The drawing under review shows one solid part. Ordinate dimensions are in mm from its lowest x, y, z. A direction names the side the tool comes from. Round coordinates to 2 decimals unless told otherwise and drop trailing zeros. Write each loop counter-clockwise with the first axis right and the second up, starting at its lowest first coordinate (ties: lowest second). Pieces come first, ordered by that corner, then holes.
Item 1: Add section D-D (y = 2.5). Give the boundary of the cut face in (x, z).
Item 2: Draft analysis for pull direction Z (two halves, no side actions). For the marked faces 1, 2 and 3, state which applies: +Z half, -Z half, draft (parallel to the pull), parting line (faces both ways), or undercut.
Item 3: Clearance check with flat-ended pins moving along their axes: pin 1 Ø7.5 at (x, z) = (19.5, 16) entering from -Y; pin 2 Ø6 at (x, y) = (36, 8.5) entering from +Z. State where each tip first meets the part, or that it passes through.
Item 4: To check wall thickness, follow L1, parallel to Y at x = 37.5, z = 1.5; L2, parallel to Y at x = 4, z = 6.25; L3, parallel to Z at x = 32.5, y = 1.5. State the ranges of each line that lie inside material, in increasing order.
Item 5: Add section C-C (x = 57.5). Give the boundary of the cut face in (y, z).
Item 6: Machinability: for the marked faces 4 and 5, which of the approach directions +Z, -Z, +X, -X, +Y, -Y give a long, thin tool a straight path to every point of the face, cutting with its end or side? Answer none if there is none.
Item 7: Add section A-A (y = 17.5). Give the boundary of the cut face in (x, z).
Item 8: Add section B-B (z = 11). Give the boundary of the cut face in (x, y), plus the area to 3 significant figures.
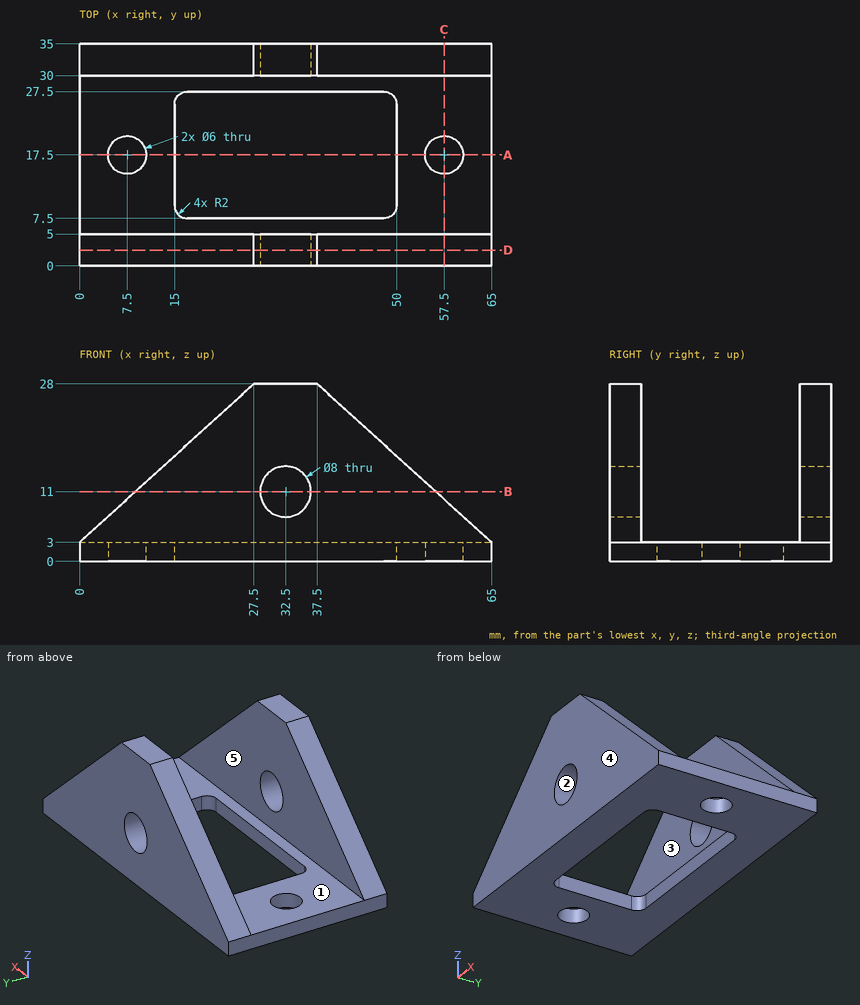
Numbers:
1. outline: (0, 0) - (65, 0) - (65, 3) - (37.5, 28) - (27.5, 28) - (0, 3) - close; hole circle Ø8 at (32.5, 11)
2. face 1: +Z half
2. face 2: undercut
2. face 3: draft
3. pin 1: stops at y = 0
3. pin 2: stops at z = 3
4. L1: y = 0 to 7.5, 27.5 to 35
4. L2: y = 0 to 5, 30 to 35
4. L3: z = 0 to 7, 15 to 28
5. outline: (0, 0) - (14.5, 0) - (14.5, 3) - (5, 3) - (5, 9.82) - (0, 9.82) - close; (20.5, 0) - (35, 0) - (35, 9.82) - (30, 9.82) - (30, 3) - (20.5, 3) - close
6. face 4: +Z, -Z, +X, -X, -Y
6. face 5: +Z, +X, -X
7. outline: (0, 0) - (4.5, 0) - (4.5, 3) - (0, 3) - close; (10.5, 0) - (15, 0) - (15, 3) - (10.5, 3) - close; (50, 0) - (54.5, 0) - (54.5, 3) - (50, 3) - close; (60.5, 0) - (65, 0) - (65, 3) - (60.5, 3) - close
8. outline: (8.8, 0) - (28.5, 0) - (28.5, 5) - (8.8, 5) - close; (8.8, 30) - (28.5, 30) - (28.5, 35) - (8.8, 35) - close; (36.5, 0) - (56.2, 0) - (56.2, 5) - (36.5, 5) - close; (36.5, 30) - (56.2, 30) - (56.2, 35) - (36.5, 35) - close
8. area: 394 mm2
